Build history of the part. All positions in model axes, mm. Face numbers are marked on the shaded views. A direction names the side the tool comes from. Give positions to 0.01 mm unless a question says otherwise; leave off trailing zeros. Write each loop counter-clockwise with the first axis right and the second up, starting at its lowest first coordinate (ties: lowest second). Pieces come first, ordered by that corner, then holes. Notation, with made-up numbers: (31, 68.5) -> (83, 68.5) arc R12 ccw to (83, 80.5) -> close; hole circle Ø3 at (-36, 80). An arc over 180 degrees is marked (long way). Put each result on its own line as item: value. Start each with the question number.
Item 1: Drill centre lines: line 1 along Y through (x, z) = (-12.5, 7.75); line 2 along X through (y, z) = (-1, 0.75); line 3 along Y through (x, z) = (-40.5, 2). Where is each one in solid material? Low to high.
Item 2: Slice it at C-C, the plane x = -29.5. List the corners of the cut face in (y, z).
Item 3: Slice it at A-A, the plane z = 9.25. List the corners of the cut face in (x, y).
Item 4: Slice it at B-B, the plane y = -9.5. List the corners of the cut face in (x, z), plus the area to 3 significant figures.
Item 5: Two-plate mould, pull along X, no slides. Class the marked faces 4 and 5: pulls with the +X half, pulls with the -X half, needs draft (parallel to the pull), parting line crosses it, or undercut.
Item 6: Slice it at D-D, the plane z = -1.25. List the corners of the cut face in (x, y).
Item 7: Flat gauge pins, fed straight in: pin 1 Ø0.5 at (x, z) = (-47.5, 8) entering from -Y; pin 2 Ø3.5 at (x, z) = (-3.5, 2.5) entering from +Y; pin 3 Ø12 at (x, y) = (-6.5, 5.5) entering from +Z; pin 4 Ø12 at (x, y) = (-43, -6.5) entering from +Z. Where does each tip first touch, or does it go through?
Item 8: Tool access for the marked faces 1, 2 and 3: list every direction of +Z, -Z, +X, -X, +Y, -Y with a clear straight run to the whole face (end or side of a thin tool).
```python
from build123d import *

# Parameters (mm, degrees)
BOSS_EXTRUDE1_DEPTH = 19
BOSS_EXTRUDE2_DEPTH = 2
BOSS_EXTRUDE3_DEPTH = 4.5
SKETCH4_W           = 4.75
SKETCH4_H           = 6
SKETCH4_W_2         = 14.25
SKETCH4_H_2         = 16
CUT_EXTRUDE1_DEPTH  = 49.452157546
SKETCH5_W           = 7
SKETCH5_H           = 12
CUT_EXTRUDE2_DEPTH  = 49.452157546
FILLET1_R           = 1
SKETCH6_R           = 1.25
BOSS_EXTRUDE4_DEPTH = 3
BOSS_EXTRUDE7_DEPTH = 8
FILLET2_R           = 2
SKETCH9_R           = 1.252428217
CUT_EXTRUDE3_DEPTH  = 10


with BuildPart() as part:
    # Sketch1 → Boss-Extrude1 (new body)
    with BuildSketch(Plane.XY):
        with BuildLine():
            Line((-34.384444189, 18.719216619), (-7.984444189, 18.719216619))
            ThreePointArc((-7.984444189, 18.719216619), (7.265555811, 3.469216619), (-7.984444189, -11.780783381))
            Line((-7.984444189, -11.780783381), (-34.384444189, -11.780783381))
            ThreePointArc((-34.384444189, -11.780783381), (-49.634444189, 3.469216619), (-34.384444189, 18.719216619))
        make_face()
        with BuildLine():
            Line((-34.384444189, 17.219216619), (-7.984444189, 17.219216619))
            ThreePointArc((-7.984444189, 17.219216619), (5.765555811, 3.469216619), (-7.984444189, -10.280783381))
            Line((-7.984444189, -10.280783381), (-34.384444189, -10.280783381))
            ThreePointArc((-34.384444189, -10.280783381), (-48.134444189, 3.469216619), (-34.384444189, 17.219216619))
        make_face(mode=Mode.SUBTRACT)
    extrude(amount=BOSS_EXTRUDE1_DEPTH)



with BuildPart() as body_2:
    # Sketch2 → Boss-Extrude2 (new body)
    with BuildSketch(Plane(origin=(0, 0, 0), x_dir=(-1, 0, 0), z_dir=(0, 0, -1))):
        with BuildLine():
            Line((34.384444189, -11.780783381), (7.984444189, -11.780783381))
            ThreePointArc((7.984444189, -11.780783381), (-7.265555811, 3.469216619), (7.984444189, 18.719216619))
            Line((7.984444189, 18.719216619), (34.384444189, 18.719216619))
            ThreePointArc((34.384444189, 18.719216619), (49.634444189, 3.469216619), (34.384444189, -11.780783381))
        make_face()
    extrude(amount=BOSS_EXTRUDE2_DEPTH)


with BuildPart() as part_1:
    add(part.part)

    add(body_2.part)  # Boss-Extrude3 merges body 2
    # Sketch3 → Boss-Extrude3 (add)
    with BuildSketch(Plane.XY):
        with BuildLine():
            Line((-22.664695889, -3.430783381), (-33.184444189, -3.430783381))
            Line((-33.184444189, -3.430783381), (-33.184444189, 10.369216619))
            Line((-33.184444189, 10.369216619), (-19.704192488, 10.369216619))
            Line((-19.704192488, 10.369216619), (-9.184444189, 10.369216619))
            Line((-9.184444189, 10.369216619), (-9.184444189, 8.469216619))
            Line((-9.184444189, 8.469216619), (4.663184056, 8.469216619))
            ThreePointArc((4.663184056, 8.469216619), (-0.337155761, 14.715615149), (-7.984444189, 17.069308538))
            Line((-7.984444189, 17.069308538), (-34.384444189, 17.069308538))
            ThreePointArc((-34.384444189, 17.069308538), (-47.984536108, 3.469216619), (-34.384444189, -10.1308753))
            Line((-34.384444189, -10.1308753), (-7.984444189, -10.1308753))
            ThreePointArc((-7.984444189, -10.1308753), (-0.337155761, -7.777181911), (4.663184056, -1.530783381))
            Line((4.663184056, -1.530783381), (-9.184444189, -1.530783381))
            Line((-9.184444189, -1.530783381), (-9.184444189, -3.430783381))
            Line((-9.184444189, -3.430783381), (-19.704192488, -3.430783381))
            Line((-19.704192488, -3.430783381), (-22.664695889, -3.430783381))
        make_face()
    extrude(amount=BOSS_EXTRUDE3_DEPTH)

    # Sketch4 → Cut-Extrude1 (cut, through all)
    with BuildSketch(Plane.ZY.offset(9.184444189)):
        with Locations((2.375, 3.469216619)):
            Rectangle(SKETCH4_W, SKETCH4_H)
        with Locations((11.875, 3.469216619)):
            Rectangle(SKETCH4_W_2, SKETCH4_H_2)
    extrude(amount=-CUT_EXTRUDE1_DEPTH, mode=Mode.SUBTRACT)

    # Sketch5 → Cut-Extrude2 (cut, through all)
    with BuildSketch(Plane(origin=(-33.184444189, 0, 0), x_dir=(0, 0, -1), z_dir=(1, 0, 0))):
        with Locations((-8, 3.469216619)):
            Rectangle(SKETCH5_W, SKETCH5_H)
    extrude(amount=-CUT_EXTRUDE2_DEPTH, mode=Mode.SUBTRACT)

    # Fillet1
    fillet1_edges = [part_1.edges().sort_by_distance(p)[0] for p in [
        (-47.580403151, -2.530783381, 11.5),
        (-47.580403151, 9.469216619, 11.5),
        (-47.580403151, 9.469216619, 4.5),
        (-47.580403151, -2.530783381, 4.5),
    ]]
    fillet(fillet1_edges, radius=FILLET1_R)

    # Sketch6 → Boss-Extrude4 (add)
    with BuildSketch(Plane(origin=(0, 0, -2), x_dir=(-1, 0, 0), z_dir=(0, 0, -1))):
        with BuildLine():
            ThreePointArc((47.662715914, -4.030783381), (49.634444189, 3.469216619), (47.662715914, 10.969216619))
            Line((47.662715914, 10.969216619), (-5.293827536, 10.969216619))
            ThreePointArc((-5.293827536, 10.969216619), (-7.265555811, 3.469216619), (-5.293827536, -4.030783381))
            Line((-5.293827536, -4.030783381), (47.662715914, -4.030783381))
        make_face()
        with Locations((21.184444189, 3.469216619)):
            Circle(SKETCH6_R, mode=Mode.SUBTRACT)
    extrude(amount=BOSS_EXTRUDE4_DEPTH)

    # Sketch10 → Boss-Extrude7 (add)
    with BuildSketch(Plane(origin=(0, 0, -2), x_dir=(-1, 0, 0), z_dir=(0, 0, -1))):
        with BuildLine():
            Line((-5.293827536, -4.030783381), (47.662715914, -4.030783381))
            ThreePointArc((47.662715914, -4.030783381), (46.201857789, -6.169830834), (44.400057001, -8.030783381))
            Line((44.400057001, -8.030783381), (-2.031168623, -8.030783381))
            ThreePointArc((-2.031168623, -8.030783381), (-3.832969412, -6.169830834), (-5.293827536, -4.030783381))
        make_face()
        with BuildLine():
            Line((-5.293827536, 10.969216619), (47.662715914, 10.969216619))
            ThreePointArc((47.662715914, 10.969216619), (46.201857789, 13.108264072), (44.400057001, 14.969216619))
            Line((44.400057001, 14.969216619), (-2.031168623, 14.969216619))
            ThreePointArc((-2.031168623, 14.969216619), (-3.832969412, 13.108264072), (-5.293827536, 10.969216619))
        make_face()
    extrude(amount=BOSS_EXTRUDE7_DEPTH)

    # Fillet2
    fillet2_edges = [part_1.edges().sort_by_distance(p)[0] for p in [
        (6.200927538, 0.469216619, 0),
        (6.200927538, 6.469216619, 0),
        (6.200927538, 6.469216619, 4.75),
        (6.200927538, 0.469216619, 4.75),
    ]]
    fillet(fillet2_edges, radius=FILLET2_R)

    # Sketch9 → Cut-Extrude3 (cut)
    with BuildSketch(Plane(origin=(0, 0, -2), x_dir=(-1, 0, 0), z_dir=(0, 0, -1))):
        with Locations((21.184444189, 3.469216619)):
            Circle(SKETCH9_R)
    extrude(amount=-CUT_EXTRUDE3_DEPTH, mode=Mode.SUBTRACT)


solid = part_1.part
```
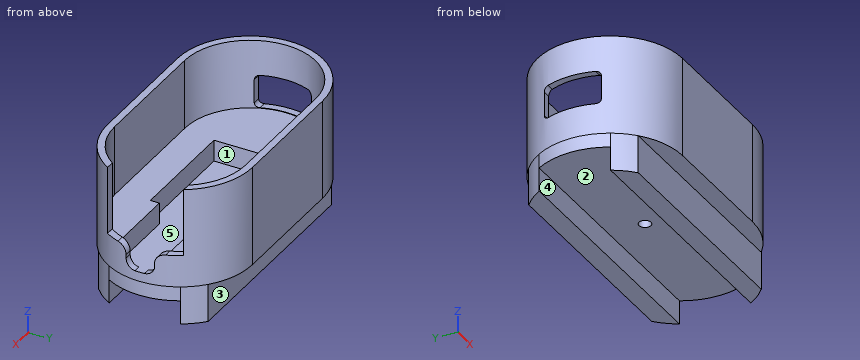
Values follow:
1. line 1: -11.78 to -10.28, 17.22 to 18.72
1. line 2: -48.96 to -47.39, -47.23 to -33.18, 5.02 to 6.6
1. line 3: -10.5 to -8.85, -8.68 to 15.62, 15.78 to 17.44
2. outline: (-11.78, -2) -> (-8.03, -2) -> (-8.03, -10) -> (-4.03, -10) -> (-4.03, -5) -> (10.97, -5) -> (10.97, -10) -> (14.97, -10) -> (14.97, -2) -> (18.72, -2) -> (18.72, 19) -> (17.22, 19) -> (17.22, 0) -> (17.07, 0) -> (17.07, 4.5) -> (10.37, 4.5) -> (10.37, 0) -> (-3.43, 0) -> (-3.43, 4.5) -> (-10.13, 4.5) -> (-10.13, 0) -> (-10.28, 0) -> (-10.28, 19) -> (-11.78, 19) -> close
3. outline: (-48.4, -2.53) arc R15.25 ccw to (-34.38, -11.78) -> (-7.98, -11.78) arc R15.25 ccw to (5, -4.53) -> (3.2, -4.53) arc R13.75 cw to (-7.98, -10.28) -> (-34.38, -10.28) arc R13.75 cw to (-46.76, -2.53) -> close; (-48.4, 9.47) -> (-46.76, 9.47) arc R13.75 cw to (-34.38, 17.22) -> (-7.98, 17.22) arc R13.75 cw to (3.2, 11.47) -> (5, 11.47) arc R15.25 ccw to (-7.98, 18.72) -> (-34.38, 18.72) arc R15.25 ccw to start
4. outline: (-42.41, -2) -> (0.04, -2) -> (0.04, 19) -> (-3.42, 19) -> (-3.42, 0) -> (-3.89, 0) -> (-3.89, 4.5) -> (-38.48, 4.5) -> (-38.48, 0) -> (-38.95, 0) -> (-38.95, 19) -> (-42.41, 19) -> close
4. area: 372 mm2
5. face 4: needs draft
5. face 5: undercut
6. outline: (-34.38, -11.78) -> (-7.98, -11.78) arc R15.25 ccw to (-7.98, 18.72) -> (-34.38, 18.72) arc R15.25 ccw to start; hole circle Ø2.5 at (-21.18, 3.47)
7. pin 1: y = -4.72
7. pin 2: y = 18.47
7. pin 3: z = 4.5
7. pin 4: z = 19
8. face 1: +Z
8. face 2: -Z, +X, -X
8. face 3: -Z, +X, -X, +Y
